```python
from build123d import *

# Parameters (mm, degrees)
SZKIC1_W                    = 18.5
SZKIC1_H                    = 15.8
DODANIE_WYCI_GNI_CIE1_DEPTH = 1.6
SZKIC2_R                    = 1.5
WYTNIJ_WYCI_GNI_CIE1_DEPTH  = 2.6
SZKIC3_W                    = 3
SZKIC3_H                    = 3
DODANIE_WYCI_GNI_CIE2_DEPTH = 1.5


with BuildPart() as part:
    # Szkic1 → Dodanie-wyciągnięcie1 (new body)
    with BuildSketch(Plane.XY):
        with Locations((9.25, 7.9)):
            Rectangle(SZKIC1_W, SZKIC1_H)
    extrude(amount=DODANIE_WYCI_GNI_CIE1_DEPTH)

    # Szkic2 → Wytnij-wyciągnięcie1 (cut, through all)
    with BuildSketch(Plane(origin=(0, 0, 0), x_dir=(-1, 0, 0), z_dir=(0, 0, -1))):
        with Locations((-2.8, 13)):
            Circle(SZKIC2_R)
        with Locations((-2.8, 2.8)):
            Circle(SZKIC2_R)
    extrude(amount=-WYTNIJ_WYCI_GNI_CIE1_DEPTH, mode=Mode.SUBTRACT)

    # Szkic3 → Dodanie-wyciągnięcie2 (add)
    with BuildSketch(Plane.XY.offset(1.6)):
        with Locations((7.5, 7.9)):
            Rectangle(SZKIC3_W, SZKIC3_H)
    extrude(amount=DODANIE_WYCI_GNI_CIE2_DEPTH)


solid = part.part
```
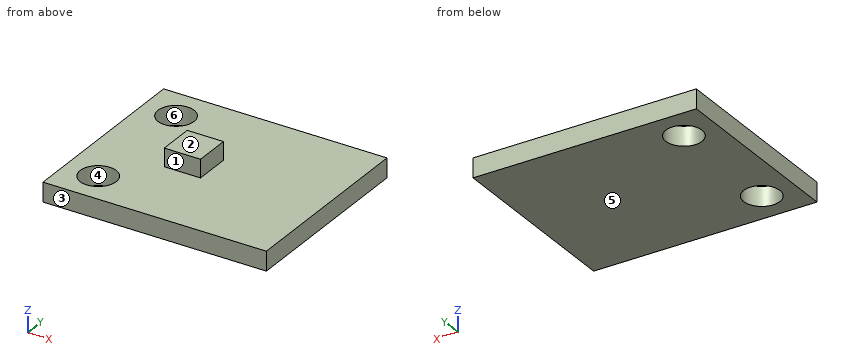
Input: part model. Units: mm. Frame: model coordinates. Face numbers are marked on the shaded views. A direction names the side the tool comes from. Give positions to 0.01 mm unless a question says otherwise; leave off trailing zeros. Order: outer loops, then holes, each group sorted by start corner. A loop starts at its lowest first (then second) coordinate and runs counter-clockwise, first axis right, second up. Notation, with made-up numbers: (57.25, 54.5) - (94.25, 54.5) arc R24 ccw to (94.25, 89.5) - close; hole circle Ø1 at (-0.5, -5.5). An arc over 180 degrees is marked (long way). Use a Markdown table: item, result.
(1) Pin query (flat end, axial travel): pin 1 (4 mm diameter, centred on x = 2.8, y = 2.8, fed in from +Z); pin 2 (4 mm diameter, centred on x = 15.5, y = 11.5, fed in from -Z); pin 3 (1.6 mm diameter, centred on x = 8, z = 2.5, fed in from +Y); pin 4 (1.6 mm diameter, centred on y = 8, z = 2.5, fed in from -X). Return the tip coordinate at first contact, or that it passes through.
Computed values:
| item | result |
|---|---|
| pin 1 | stops at z = 1.6 |
| pin 2 | stops at z = 0 |
| pin 3 | stops at y = 9.4 |
| pin 4 | stops at x = 6 |
(2) Section query A-A (y = 13). Output: boundary loops of the cut face in (x, z), then the cut area to 3 significant figures.
Computed values:
| item | result |
|---|---|
| outline | (0, 0) - (1.3, 0) - (1.3, 1.6) - (0, 1.6) - close; (4.3, 0) - (18.5, 0) - (18.5, 1.6) - (4.3, 1.6) - close |
| area | 24.8 mm2 |
(3) Section query C-C (z = 1.4). Output: boundary loops of the cut face in (x, y).
Computed values:
| item | result |
|---|---|
| outline | (0, 0) - (18.5, 0) - (18.5, 15.8) - (0, 15.8) - close; hole circle Ø3 at (2.8, 2.8); hole circle Ø3 at (2.8, 13) |
(4) Line query: line 1 (Y direction, x = 2.8, z = 1.35); line 2 (Y direction, x = 3.5, z = 1.2); line 3 (Z direction, x = 16.25, y = 5.75). Output: solid intervals per line, ascending. Write a range as from..to.
Computed values:
| item | result |
|---|---|
| line 1 | y = 0..1.3, 4.3..11.5, 14.5..15.8 |
| line 2 | y = 0..1.47, 4.13..11.67, 14.33..15.8 |
| line 3 | z = 0..1.6 |
(5) Section query B-B (x = 2.8). Output: boundary loops of the cut face in (y, z), then the cut area to 3 significant figures.
Computed values:
| item | result |
|---|---|
| outline | (0, 0) - (1.3, 0) - (1.3, 1.6) - (0, 1.6) - close; (4.3, 0) - (11.5, 0) - (11.5, 1.6) - (4.3, 1.6) - close; (14.5, 0) - (15.8, 0) - (15.8, 1.6) - (14.5, 1.6) - close |
| area | 15.7 mm2 |
(6) Section query D-D (y = 7). Output: boundary loops of the cut face in (x, z), then the cut area to 3 significant figures.
Computed values:
| item | result |
|---|---|
| outline | (0, 0) - (18.5, 0) - (18.5, 1.6) - (9, 1.6) - (9, 3.1) - (6, 3.1) - (6, 1.6) - (0, 1.6) - close |
| area | 34.1 mm2 |
(7) Draft query along Y for the marked faces 3, 4, 5 and 6. Return one class per face: released by +Y, released by -Y, zero draft, split by the parting line, or undercut.
Computed values:
| item | result |
|---|---|
| face 3 | released by -Y |
| face 4 | undercut |
| face 5 | zero draft |
| face 6 | undercut |
(8) Access query for the marked faces 1 and 2. Directions: +Z, -Z, +X, -X, +Y, -Y. A direction counts if a zero-diameter tool reaches every point of the face in a straight line with its end or side. Return the directions, or none.
Computed values:
| item | result |
|---|---|
| face 1 | +Z, +X, -X, -Y |
| face 2 | +Z, +X, -X, +Y, -Y |
